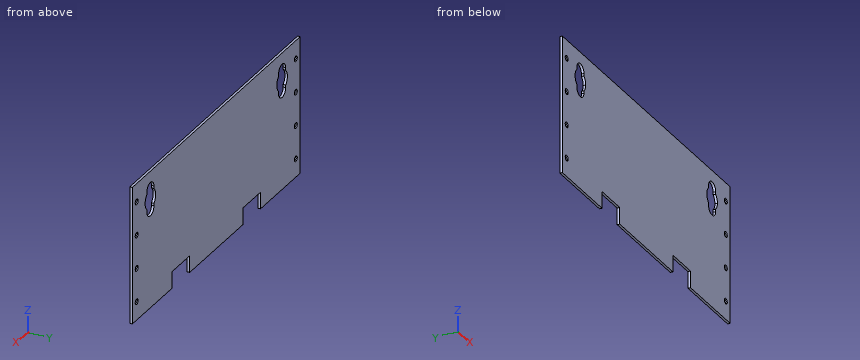
from build123d import *

# Parameters (mm, degrees)
SKETCH_W        = 190
SKETCH_H        = 82
SKETCH_R        = 1.65
PAD_DEPTH       = 0.75
PAD_DEPTH_BACK  = 0.75
SKETCH001_W     = 20
SKETCH001_H     = 10
POCKET_DEPTH    = 1.501
POCKET001_DEPTH = 1.501
SKETCH003_R     = 6
POCKET002_DEPTH = 1.501


with BuildPart() as part:
    # Sketch → Pad (new body, two sides)
    with BuildSketch(Plane.XZ) as pad_sk:
        Rectangle(SKETCH_W, SKETCH_H)
        with Locations((90, 30)):
            Circle(SKETCH_R, mode=Mode.SUBTRACT)
        with Locations((90, 10)):
            Circle(SKETCH_R, mode=Mode.SUBTRACT)
        with Locations((90, -30)):
            Circle(SKETCH_R, mode=Mode.SUBTRACT)
        with Locations((90, -10)):
            Circle(SKETCH_R, mode=Mode.SUBTRACT)
        with Locations((-90, 30)):
            Circle(SKETCH_R, mode=Mode.SUBTRACT)
        with Locations((-90, 10)):
            Circle(SKETCH_R, mode=Mode.SUBTRACT)
        with Locations((-90, -30)):
            Circle(SKETCH_R, mode=Mode.SUBTRACT)
        with Locations((-90, -10)):
            Circle(SKETCH_R, mode=Mode.SUBTRACT)
    extrude(amount=PAD_DEPTH)
    extrude(pad_sk.sketch, amount=-PAD_DEPTH_BACK)

    # Sketch001 (on Face14 of Pad) → Pocket (cut, through all)
    with BuildSketch(Plane.XZ.offset(0.75)):
        with Locations((-40, -36)):
            Rectangle(SKETCH001_W, SKETCH001_H)
        with Locations((40, -36)):
            Rectangle(SKETCH001_W, SKETCH001_H)
    extrude(amount=-POCKET_DEPTH, mode=Mode.SUBTRACT)

    # Sketch002 (on Face5 of Pocket) → Pocket001 (cut, through all)
    with BuildSketch(Plane.XZ.offset(0.75)):
        with BuildLine():
            ThreePointArc((78.5, 30.25), (74.5, 34.25), (70.5, 30.25))
            Line((70.5, 30.25), (70.5, 18.25))
            ThreePointArc((70.5, 18.25), (74.5, 14.25), (78.5, 18.25))
            Line((78.5, 30.25), (78.5, 18.25))
        make_face()
        with BuildLine():
            ThreePointArc((-70.5, 30.25), (-74.5, 34.25), (-78.5, 30.25))
            Line((-78.5, 30.25), (-78.5, 18.25))
            ThreePointArc((-78.5, 18.25), (-74.5, 14.25), (-70.5, 18.25))
            Line((-70.5, 30.25), (-70.5, 18.25))
        make_face()
    extrude(amount=-POCKET001_DEPTH, mode=Mode.SUBTRACT)

    # Sketch003 (on Face5 of Pocket001) → Pocket002 (cut, through all)
    with BuildSketch(Plane.XZ.offset(0.75)):
        with Locations((-74.5, 24.25)):
            Circle(SKETCH003_R)
        with Locations((74.5, 24.25)):
            Circle(SKETCH003_R)
    extrude(amount=-POCKET002_DEPTH, mode=Mode.SUBTRACT)


solid = part.part
CAD build for the part. Positions are in the model's coordinates, mm. Coordinates: 2 decimals unless noted, no trailing zeros. Write each loop counter-clockwise with the first axis right and the second up, starting at its lowest first coordinate (ties: lowest second). Pieces come first, ordered by that corner, then holes. Notation, with made-up numbers: M 50.5,-19.5 L 83.5,-19.5 A23 ccw 83.5,9.5 Z; hole C -8,-27.75 d3. An arc over 180 degrees is marked long. Answer as a JSON object with one key per item and string values. Group by question number.
1) Saw through at B-B (x = 44.5). Write the cut outline in (y, z), plus the area to 3 significant figures.
2) Saw through at A-A (x = -74.5). Write the cut outline in (y, z), plus the area to 3 significant figures.
3) Wall check: line 1 (X direction, y = -0.35, z = -32); line 2 (Z direction, x = 90, y = -0.45); line 3 (Z direction, x = 35, y = -0.3). Give the ranges that are in metal, low to high. Write a range as from..to.
4) Saw through at C-C (y = -0.45). Give the number of separate pieces and of enclosed holes in the cut face, plus the area to 3 significant figures.
Values follow:
{
 "1": {"outline": "M -0.75,-31 L 0.75,-31 L 0.75,41 L -0.75,41 Z", "area": "108 mm2"},
 "2": {"outline": "M -0.75,-41 L 0.75,-41 L 0.75,14.25 L -0.75,14.25 Z; M -0.75,34.25 L 0.75,34.25 L 0.75,41 L -0.75,41 Z", "area": "93.0 mm2"},
 "3": {"line 1": "x = -95..-50, -30..30, 50..95", "line 2": "z = -41..-31.65, -28.35..-11.65, -8.35..8.35, 11.65..28.35, 31.65..41", "line 3": "z = -31..41"},
 "4": {"separate pieces": "1", "enclosed holes": "10", "area": "14,800 mm2"}
}
